```python
from build123d import *

# Parameters (mm, degrees)
BOSS_EXTRUDE3_DEPTH = 74
CUT_EXTRUDE5_DEPTH  = 74
SKETCH14_R          = 3
CUT_EXTRUDE6_DEPTH  = 74
SKETCH15_R          = 8
CUT_EXTRUDE7_DEPTH  = 13
CUT_EXTRUDE8_DEPTH  = 90
CUT_EXTRUDE10_DEPTH = 22
SKETCH20_R          = 5
CUT_EXTRUDE11_DEPTH = 22


with BuildPart() as part:
    # Sketch2 → Boss-Extrude3 (new body)
    with BuildSketch(Plane.XY):
        Polygon((0, 0), (0, 30), (16.036697248, 30), (16.036697248, -33), (-135.963302752, -33), (-135.963302752, 18), (-135.963302752, 32), (-115.963302752, 32), (-105.963302752, 32), (-105.963302752, 0), align=None)
    extrude(amount=BOSS_EXTRUDE3_DEPTH)

    # Sketch11 → Cut-Extrude5 (cut)
    with BuildSketch(Plane.XY.offset(74)):
        Polygon((-135.963302752, 11.943655514), (-135.963302752, 32), (-115.906958266, 32), align=None)
    extrude(amount=-CUT_EXTRUDE5_DEPTH, mode=Mode.SUBTRACT)

    # Sketch14 → Cut-Extrude6 (cut)
    with BuildSketch(Plane(origin=(-105.963302752, 0, 0), x_dir=(0, 0, -1), z_dir=(1, 0, 0))):
        with Locations((-61, 18)):
            Circle(SKETCH14_R)
        with Locations((-13, 18)):
            Circle(SKETCH14_R)
    extrude(amount=-CUT_EXTRUDE6_DEPTH, mode=Mode.SUBTRACT)

    # Sketch15 → Cut-Extrude7 (cut)
    with BuildSketch(Plane.ZY.offset(135.963302752)):
        with Locations((36.610721791, -4.86425639)):
            Circle(SKETCH15_R)
    extrude(amount=-CUT_EXTRUDE7_DEPTH, mode=Mode.SUBTRACT)

    # Sketch16 → Cut-Extrude8 (cut)
    with BuildSketch(Plane(origin=(0, 0, 0), x_dir=(1, 0, 0), z_dir=(0, 1, 0))):
        with BuildLine():
            Line((-86.67307708, -29), (-8.67307708, -29))
            ThreePointArc((-8.67307708, -29), (-0.67307708, -37), (-8.67307708, -45))
            Line((-8.67307708, -45), (-86.67307708, -45))
            ThreePointArc((-86.67307708, -45), (-94.67307708, -37), (-86.67307708, -29))
        make_face()
    extrude(amount=-CUT_EXTRUDE8_DEPTH, mode=Mode.SUBTRACT)

    # Sketch19 → Cut-Extrude10 (cut)
    with BuildSketch(Plane(origin=(16.036697248, 0, 0), x_dir=(0, 0, -1), z_dir=(1, 0, 0))):
        Polygon((-74, 30), (-74, 0), (-49.5, 30), align=None)
        Polygon((0, 0), (0, 30), (-24.5, 30), align=None)
    extrude(amount=-CUT_EXTRUDE10_DEPTH, mode=Mode.SUBTRACT)

    # Sketch20 → Cut-Extrude11 (cut)
    with BuildSketch(Plane(origin=(16.036697248, 0, 0), x_dir=(0, 0, -1), z_dir=(1, 0, 0))):
        with Locations(Location((-37.135567798, 16.44, 0), (0, 0, 90))):
            Circle(SKETCH20_R)
    extrude(amount=-CUT_EXTRUDE11_DEPTH, mode=Mode.SUBTRACT)


solid = part.part
```
Input: part model. Units: mm. Frame: model coordinates. A direction names the side the tool comes from. Give positions to 0.01 mm unless a question says otherwise; leave off trailing zeros. Loops run counter-clockwise (first coordinate to the right, second up) from the corner with the lowest first, then second, coordinate; pieces in that order, holes last. Notation, with made-up numbers: M -37,-24 L 21,-24 A27 ccw 21,-1 Z; hole C 79.5,70 d1. An arc over 180 degrees is marked long. Answer as CSV lines item,"result". Start each with the question number.
1. Pin query (flat end, axial travel): P1, Ø8, axis at y = 16.44, z = 37.14, coming from the +X side; P2, Ø2, axis at x = -40.5, z = 64.5, coming from the +Y side; P3, Ø13, axis at x = 6.5, z = 43, coming from the +Y side. Return the tip coordinate at first contact, or that it passes through.
2. Line query: L1, parallel to Z at x = -60.5, y = -24; L2, parallel to Y at x = -112.25, z = 13; L3, parallel to X at y = 0.5, z = 52.5. Output: solid intervals per line, ascending.
3. Section A-A on x = -64. Return loops of the section in (y, z), plus the area to 3 significant figures.
4. Section B-B on z = 13. Return loops of the section in (x, y), plus the area to 3 significant figures.
5. Reachability of faces 1 (the face through (8.13, 14.79, 61.92)), 2 (the face through (8, 30, 37)), 3 (the face through (-105.963, 16, 36)), 4 (the face through (-119.25, 15.07, 13.65)) from +Z, -Z, +X, -X, +Y, -Y: full face, straight path, thin tool, end or side. Return the list, or none.
6. Section D-D on y = 18. Return loops of the section in (x, z).
7. Section C-C on y = -24. Return loops of the section in (x, z), plus the area to 3 significant figures.
8. Pull-direction query (X, two-part tool) for faces 5 (the face through (-111, 32, 36)), 6 (the face through (-135.963, -15, 36)), 7 (the face through (-48, -16, 29)); classes: released by +X, released by -X, zero draft, split by the parting line, or undercut.
Computed values:
1,P1,"stops at x = -105.96"
1,P2,"stops at y = 0"
1,P3,"stops at y = 30"
2,L1,"z = 0 to 29, 45 to 74"
2,L2,"y = -33 to 15, 21 to 32"
2,L3,"x = -135.96 to -105.96, 0 to 16.04"
3,outline,"M -33,0 L 0,0 L 0,29 L -33,29 Z; M -33,45 L 0,45 L 0,74 L -33,74 Z"
3,area,"1,910 mm²"
4,outline,"M -135.96,-33 L 16.04,-33 L 16.04,15.92 L 0,15.92 L 0,0 L -105.96,0 L -105.96,15 L -132.91,15 L -135.96,11.94 Z; M -126.91,21 L -105.96,21 L -105.96,32 L -115.91,32 Z"
4,area,"5,890 mm²"
5,face 1,"+Z, +X, +Y"
5,face 2,"+Z, -Z, +X, +Y"
5,face 3,"+Z, -Z, +Y"
5,face 4,"-X"
6,outline,"M -129.91,0 L -105.96,0 L -105.96,10 L -129.91,10 Z; M -129.91,16 L -105.96,16 L -105.96,58 L -129.91,58 Z; M -129.91,64 L -105.96,64 L -105.96,74 L -129.91,74 Z; M 0,14.7 L 16.04,14.7 L 16.04,32.39 L 0,32.39 Z; M 0,41.89 L 16.04,41.89 L 16.04,59.3 L 0,59.3 Z"
7,outline,"M -135.96,0 L 16.04,0 L 16.04,74 L -135.96,74 Z; hole M -86.67,29 L -8.67,29 A8 ccw -8.67,45 L -86.67,45 A8 ccw Z"
7,area,"9,800 mm²"
8,face 5,"zero draft"
8,face 6,"released by -X"
8,face 7,"undercut"
